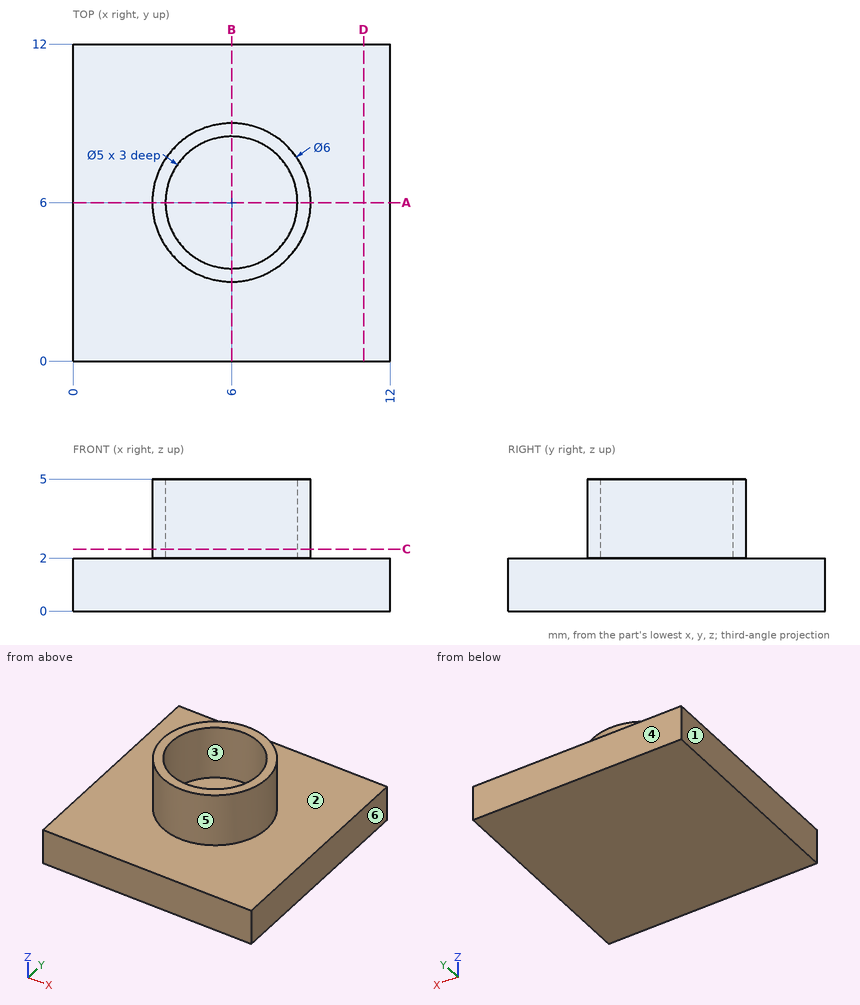
The figure shows three views and two pictorial views of one solid part (mm, origin at its lowest corner). Answer the questions. A direction names the side the tool comes from. Give positions to 0.01 mm unless a question says otherwise; leave off trailing zeros. Write each loop counter-clockwise with the first axis right and the second up, starting at its lowest first coordinate (ties: lowest second). Pieces come first, ordered by that corner, then holes. Notation, with made-up numbers: M 17.25,7 L 41.25,7 A29 cw 41.25,36 Z; hole C 88.5,-6 d3. An arc over 180 degrees is marked long. Write each question's results on one line, items separated by ' | '.
Q1. For a pull along X with two mould halves and no side action, classify the marked faces 3, 4, 5 and 6 as released by +X, released by -X, zero draft, split by the parting line, or undercut.
Output values:
face 3: undercut | face 4: zero draft | face 5: split by the parting line | face 6: released by +X
Q2. Section D-D, the plane x = 11 is taken. Write down the section's boundary in (y, z), then the cut area to 3 significant figures.
Output values:
outline: M 0,0 L 12,0 L 12,2 L 0,2 Z | area: 24.0 mm2
Q3. A tool of negligible diameter and unlimited length cuts with its end or side. For the marked faces 1 and 2, from which of +Z, -Z, +X, -X, +Y, -Y can it reach the whole face along a straight path? Write none if from no direction.
Output values:
face 1: +Z, -Z, -X, +Y, -Y | face 2: +Z
Q4. Flat-ended cylindrical pins translate along their axes: P1, Ø1.5, axis at y = 6.5, z = 3.5, coming from the +X side; P2, Ø1, axis at y = 2, z = 3, coming from the -X side; P3, Ø1.5, axis at x = 6, y = 6.5, coming from the +Z side. Find the tip coordinate at first contact, or state that the pin passes through.
Output values:
P1: x = 9 | P2: through | P3: z = 2
Q5. Section C-C, the plane z = 2.35 is taken. Write down the section's boundary in (x, y), then the cut area to 3 significant figures.
Output values:
outline: C 6,6 d6; hole C 6,6 d5 | area: 8.64 mm2
Q6. Section A-A, the plane y = 6 is taken. Write down the section's boundary in (x, z), then the cut area to 3 significant figures.
Output values:
outline: M 0,0 L 12,0 L 12,2 L 9,2 L 9,5 L 8.5,5 L 8.5,2 L 3.5,2 L 3.5,5 L 3,5 L 3,2 L 0,2 Z | area: 27.0 mm2
Q7. Consider L1, parallel to Y at x = 6, z = 4.25; L2, parallel to Z at x = 5, y = 3; L3, parallel to Y at x = 6.75, z = 3.95. Determine where each line is inside the solid, lowest interval first. Write a range as from..to.
Output values:
L1: 3..3.5, 8.5..9 | L2: 0..2 | L3: 3.1..3.62, 8.38..8.9
